Verification items for the finished model (mm, model axes). A direction names the side the tool comes from. Coordinates: 2 decimals unless noted, no trailing zeros. Write each loop counter-clockwise with the first axis right and the second up, starting at its lowest first coordinate (ties: lowest second). Pieces come first, ordered by that corner, then holes. Notation, with made-up numbers: M -39.75,49.25 L -30.75,49.25 A19 ccw -30.75,65.25 Z; hole C 19,64 d2. An arc over 180 degrees is marked long. One line per item, written item: value.
```python
from build123d import *

# Parameters (mm, degrees)
EXTRUDE_1_DEPTH          = 37.5
SKETCH_4_W               = 2.5
SKETCH_4_H               = 30
CUT_EXTRUDE_2_DEPTH      = 33.5
CUT_EXTRUDE_3_DEPTH      = 44.084219849
CUT_EXTRUDE_3_DEPTH_BACK = 33.5
CUT_EXTRUDE_4_DEPTH      = 33
SKETCH_12_W              = 9
SKETCH_12_H              = 30
CUT_EXTRUDE_7_DEPTH      = 33
CUT_EXTRUDE_8_REACH      = 49.765
SKETCH_16_R              = 7.5
CHAMFER_2_SIZE           = 2


with BuildPart() as part:
    # 草图1 → 凸台-拉伸1 (new body)
    with BuildSketch(Plane(origin=(0, 0, 0), x_dir=(1, 0, 0), z_dir=(0, 1, 0))):
        Polygon((13, -15), (15, -13), (15, 13), (13, 15), (-13, 15), (-15, 13), (-15, -13), (-13, -15), align=None)
    extrude(amount=EXTRUDE_1_DEPTH)

    # 草图4 → 切除-拉伸2 (cut)
    with BuildSketch(Plane(origin=(0, 37.5, 0), x_dir=(1, 0, 0), z_dir=(0, 1, 0))):
        with Locations((-11.75, 0)):
            Rectangle(SKETCH_4_W, SKETCH_4_H)
    extrude(amount=-CUT_EXTRUDE_2_DEPTH, mode=Mode.SUBTRACT)

    # 草图9 → 切除-拉伸3 (cut, two sides: drawn at the far end of the back side and taken through both)
    with BuildSketch(Plane(origin=(0, 37.5, 0), x_dir=(1, 0, 0), z_dir=(0, 1, 0)).offset(-CUT_EXTRUDE_3_DEPTH_BACK)):
        Polygon((-13, -15), (-13, 15), (-15, 13), (-15, -13), align=None)
    extrude(amount=CUT_EXTRUDE_3_DEPTH + CUT_EXTRUDE_3_DEPTH_BACK, mode=Mode.SUBTRACT)

    # 草图11 → 切除-拉伸4 (cut)
    with BuildSketch(Plane(origin=(0, 37.5, 0), x_dir=(1, 0, 0), z_dir=(0, 1, 0))):
        Polygon((10.5, -15), (10.5, 15), (13, 15), (15, 13), (15, -13), (13, -15), align=None)
    extrude(amount=-CUT_EXTRUDE_4_DEPTH, mode=Mode.SUBTRACT)

    # 草图12 → 切除-拉伸7 (cut)
    with BuildSketch(Plane(origin=(0, 37.5, 0), x_dir=(1, 0, 0), z_dir=(0, 1, 0))):
        Rectangle(SKETCH_12_W, SKETCH_12_H)
    extrude(amount=-CUT_EXTRUDE_7_DEPTH, mode=Mode.SUBTRACT)

    # 切除-拉伸8: up to this face of the body (flat: up to its plane)
    cut_extrude_8_end = Plane(part.part.faces().sort_by_distance((10.5, 21, 0))[0])
    # 草图16 → 切除-拉伸8 (cut, up to the picked face)
    with BuildSketch(Plane.ZY.offset(10.5), mode=Mode.PRIVATE) as cut_extrude_8_sk1:
        with Locations((0, 25)):
            Circle(SKETCH_16_R)
    cut_extrude_8_tool1 = split(extrude(cut_extrude_8_sk1.sketch, amount=-CUT_EXTRUDE_8_REACH, mode=Mode.PRIVATE), bisect_by=cut_extrude_8_end, keep=Keep.BOTH, mode=Mode.PRIVATE)
    add(cut_extrude_8_tool1.solids().sort_by(Axis((-10.5, 25, 0), (1, 0, 0)))[0], mode=Mode.SUBTRACT)

    # 倒角2
    chamfer_2_edges = [part.edges().sort_by_distance(p)[0] for p in [
        (-7.5, 37.5, 15),
        (-7.5, 37.5, -15),
        (7.5, 37.5, -15),
        (7.5, 37.5, 15),
    ]]
    chamfer(chamfer_2_edges, length=CHAMFER_2_SIZE)


solid = part.part
```
Item 1: Go/stop test with flat-tipped pins: P1, Ø8, axis at y = 18, z = 0.5, coming from the +X side; P2, Ø1.3, axis at x = 12, z = -7, coming from the +Y side; P3, Ø4, axis at y = 11, z = 10.5, coming from the -X side. Record where each tip stops, or that it passes through.
The answers:
P1: stops at x = 10.5
P2: stops at y = 4.5
P3: stops at x = -10.5
Item 2: Cross-section at C-C, the plane x = 5.5. Enter the section's corners in (y, z), and give its area (3 significant figures).
The answers:
outline: M 0,-15 L 35.5,-15 L 37.5,-13 L 37.5,13 L 35.5,15 L 0,15 Z; hole C 25,0 d15
area: 944 mm²
Item 3: Scan lines: line 1 (Y direction, x = -7.7, z = 0); line 2 (X direction, y = 19, z = -10.5); line 3 (Y direction, x = -2, z = -6.5). Record each from-to range of solid material in increasing order.
The answers:
line 1: y = 0 to 17.5, 32.5 to 37.5
line 2: x = -10.5 to -4.5, 4.5 to 10.5
line 3: y = 0 to 4.5
Item 4: Access from +Z, -Z, +X, -X, +Y, -Y to the whole of each face (thin tool, end or side, straight path). Record for faces 1 (the face through (-4.5, 18, 4)), 2 (the face through (-15, 2, 0)), 3 (the face through (10.5, 18, 4)).
The answers:
face 1: +Z, -Z, +Y
face 2: +Z, -Z, -X, +Y, -Y
face 3: +Z, -Z, +X, +Y
Item 5: Cross-section at A-A, the plane z = 0. Enter the section's corners in (x, y), and give its area (3 significant figures).
The answers:
outline: M -15,0 L 15,0 L 15,4.5 L 10.5,4.5 L 10.5,17.5 L 4.5,17.5 L 4.5,4.5 L -4.5,4.5 L -4.5,17.5 L -10.5,17.5 L -10.5,4 L -15,4 Z; M -10.5,32.5 L -4.5,32.5 L -4.5,37.5 L -10.5,37.5 Z; M 4.5,32.5 L 10.5,32.5 L 10.5,37.5 L 4.5,37.5 Z
area: 349 mm²
Item 6: Draft check along X on faces 4 (the face through (-13, 4, 0)), 5 (the face through (14, 2, -14)), 6 (the face through (4.5, 18, 4)). Enter one of: released by +X, released by -X, zero draft, split by the parting line, or undercut.
The answers:
face 4: zero draft
face 5: released by +X
face 6: undercut
Item 7: Cross-section at D-D, the plane y = 34.5. Enter the section's corners in (x, z).
The answers:
outline: M -10.5,-15 L -4.5,-15 L -4.5,15 L -10.5,15 Z; M 4.5,-15 L 10.5,-15 L 10.5,15 L 4.5,15 Z
Item 8: Cross-section at B-B, the plane y = 25. Enter the section's corners in (x, z), and give its area (3 significant figures).
The answers:
outline: M -10.5,-15 L -4.5,-15 L -4.5,-7.5 L -10.5,-7.5 Z; M -10.5,7.5 L -4.5,7.5 L -4.5,15 L -10.5,15 Z; M 4.5,-15 L 10.5,-15 L 10.5,-7.5 L 4.5,-7.5 Z; M 4.5,7.5 L 10.5,7.5 L 10.5,15 L 4.5,15 Z
area: 180 mm²
